For this review, take the finished solid that the model builds, in its own axes (mm). Face numbers are marked on the shaded views. A direction names the side the tool comes from. Round coordinates to 2 decimals unless told otherwise and drop trailing zeros. Order: outer loops, then holes, each group sorted by start corner. A loop starts at its lowest first (then second) coordinate and runs counter-clockwise, first axis right, second up. Notation, with made-up numbers: (4.5, 62.25) - (49.5, 62.25) arc R17 cw to (49.5, 79.25) - close; hole circle Ø2 at (-29, 42). An arc over 180 degrees is marked (long way). One line per item, written item: value.
```python
from build123d import *


with BuildPart() as part:
    # Sketch2 → Revolve6 (revolve)
    with BuildSketch(Plane.XY, mode=Mode.PRIVATE) as revolve6_sk:
        Polygon((1600, 50), (1600, 25), (1800, 25), (1800, 0), (400, 0), (400, 200), (0, 200), (0, 250), (400, 250), (400, 400), (600, 400), (600, 250), (800, 250), (800, 200), (1000, 200), (1000, 150), (1200, 150), (1200, 100), (1400, 100), (1400, 50), align=None)
    revolve(revolve6_sk.sketch.rotate(Axis((0, 0, 0), (1, 0, 0)), 90), axis=Axis((0, 0, 0), (1, 0, 0)))  # turned: the seam where the file's is


solid = part.part
```
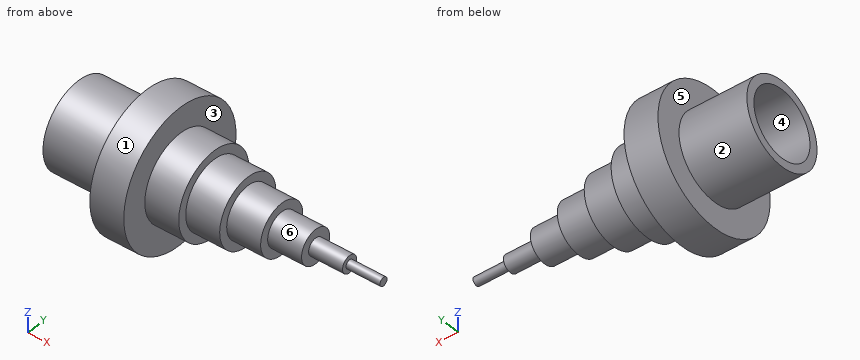
Item 1: Take a section at C-C (z = 171). Write out the cut boundary in (x, y).
Returned:
outline: (0, -182.37) - (400, -182.37) - (400, -361.61) - (600, -361.61) - (600, -182.37) - (800, -182.37) - (800, -103.73) - (1000, -103.73) - (1000, 103.73) - (800, 103.73) - (800, 182.37) - (600, 182.37) - (600, 361.61) - (400, 361.61) - (400, 182.37) - (0, 182.37) - (0, 103.73) - (400, 103.73) - (400, -103.73) - (0, -103.73) - close
Item 2: Take a section at B-B (x = 247). Write out the cut boundary in (y, z).
Returned:
outline: circle Ø500 at (0, 0); hole circle Ø400 at (0, 0)
Item 3: The part is to be moulded in two halves that separate along Y. For the marked faces 4, 5 and 6, say which applies: +Y half, -Y half, draft (parallel to the pull), parting line (faces both ways), or undercut.
Returned:
face 4: undercut
face 5: draft
face 6: parting line
Item 4: For P1, Ø3, axis at y = 168, z = -271.5, coming from the +X side; P2, Ø12, axis at x = 1088, y = -11.5, coming from the +Z side; P3, Ø12, axis at x = 771, z = -188.5, coming from the -Y side, all flat-tipped, find the tip position at first contact; note any pin that passes through.
Returned:
P1: x = 600
P2: z = 149.9
P3: y = -170.86
Item 5: Machinability: for the marked faces 1, 2 and 3, which of the approach directions +Z, -Z, +X, -X, +Y, -Y give a long, thin tool a straight path to every point of the face, cutting with its end or side? Answer none if there is none.
Returned:
face 1: +X, -X
face 2: -X
face 3: +X
Item 6: Wall thickness on line 1 (Y direction, x = 293.5, z = 0); line 2 (X direction, y = -69.5, z = 344); line 3 (Z direction, x = 102, y = -145.5): over which ranges is each line inside the solid? List them lowest first.
Returned:
line 1: -250 to -200, 200 to 250
line 2: 400 to 600
line 3: -203.3 to -137.22, 137.22 to 203.3
Item 7: Take a section at A-A (y = -74.5). Write out the cut boundary in (x, z), plus the area to 3 significant figures.
Returned:
outline: (0, -238.64) - (400, -238.64) - (400, -393) - (600, -393) - (600, -238.64) - (800, -238.64) - (800, -185.61) - (1000, -185.61) - (1000, -130.19) - (1200, -130.19) - (1200, -66.71) - (1400, -66.71) - (1400, 66.71) - (1200, 66.71) - (1200, 130.19) - (1000, 130.19) - (1000, 185.61) - (800, 185.61) - (800, 238.64) - (600, 238.64) - (600, 393) - (400, 393) - (400, 238.64) - (0, 238.64) - (0, 185.61) - (400, 185.61) - (400, -185.61) - (0, -185.61) - close
area: 448,000 mm^2
Item 8: Take a section at D-D (x = 731.5). Write out the cut boundary in (y, z).
Returned:
outline: circle Ø500 at (0, 0)
